```python
from build123d import *

# Parameters (mm, degrees)
SKETCH_1_R          = 34
EXTRUDE_1_DEPTH     = 29
SKETCH_2_R          = 25
CUT_EXTRUDE_1_DEPTH = 5
CUT_EXTRUDE_START   = -5
SKETCH_3_R          = 25
CUT_EXTRUDE_2_DEPTH = 5
CUT_EXTRUDE_3_DEPTH = 10
SKETCH_5_R          = 1.4
CUT_EXTRUDE_4_DEPTH = 54.74011537


with BuildPart() as part:
    # 草图1 → 凸台-拉伸1 (new body)
    with BuildSketch(Plane.XY):
        with Locations(Location((0, 0, 0), (0, 0, 180))):
            Circle(SKETCH_1_R)
    extrude(amount=EXTRUDE_1_DEPTH)

    # 草图2 → 切除-拉伸1 (cut)
    with BuildSketch(Plane.XY.offset(29)):
        Circle(SKETCH_2_R)
    extrude(amount=-CUT_EXTRUDE_1_DEPTH, mode=Mode.SUBTRACT)

    # 草图3 → 切除-拉伸2 (cut)
    with BuildSketch(Plane(origin=(0, 0, 0), x_dir=(-1, 0, 0), z_dir=(0, 0, -1)).offset(CUT_EXTRUDE_START)):
        with Locations(Location((0, 0, 0), (0, 0, 180))):
            Circle(SKETCH_3_R)
    extrude(amount=CUT_EXTRUDE_2_DEPTH, mode=Mode.SUBTRACT)

    # 草图4 → 切除-拉伸3 (cut)
    with BuildSketch(Plane(origin=(0, 0, 5), x_dir=(-1, 0, 0), z_dir=(0, 0, -1))):
        Polygon((2.352778868, -3.142891174), (3.898213032, 0.466120682), (1.545434164, 3.609011856), (-2.352778868, 3.142891174), (-3.898213032, -0.466120682), (-1.545434164, -3.609011856), align=None)
    extrude(amount=-CUT_EXTRUDE_3_DEPTH, mode=Mode.SUBTRACT)

    # 草图5 → 切除-拉伸4 (cut, through all)
    with BuildSketch(Plane.XY.offset(24)):
        Circle(SKETCH_5_R)
    extrude(amount=-CUT_EXTRUDE_4_DEPTH, mode=Mode.SUBTRACT)


solid = part.part
```
The listing builds one solid part. Answer for the finished solid, in the listing's coordinates (mm). A direction names the side the tool comes from. Give positions to 0.01 mm unless a question says otherwise; leave off trailing zeros. Order: outer loops, then holes, each group sorted by start corner. A loop starts at its lowest first (then second) coordinate and runs counter-clockwise, first axis right, second up. Notation, with made-up numbers: (89.25, 9.5) -> (140.25, 9.5) arc R12 ccw to (140.25, 28.5) -> close; hole circle Ø10 at (-24.5, 21.5). An arc over 180 degrees is marked (long way). One line per item, written item: value.
1) Find the intervals of material crossed by line 1 (Y direction, x = 0, z = 20.25); line 2 (Y direction, x = 0, z = 3.9); line 3 (Z direction, x = -15, y = 1), in increasing order.
Reported:
line 1: y = -34 to -1.4, 1.4 to 34
line 2: y = -34 to -25, 25 to 34
line 3: z = 5 to 24
2) A tool of negligible diameter and unlimited length cuts with its end or side. For faces 1 (the flat face through (-2.738, 2.016, 9.93)), 2 (the cylindrical face through (23.846, 7.509, 26.535)), 3 (the cylindrical face through (-1.4, 0.06, 19.56)), from which of +Z, -Z, +X, -X, +Y, -Y can it reach the whole face along a straight path? Write none if from no direction.
Reported:
face 1: -Z
face 2: +Z
face 3: +Z, -Z
3) Find section D-D, the plane x = 16. Determine the outline of the cut face in (y, z).
Reported:
outline: (-30, 0) -> (-19.21, 0) -> (-19.21, 5) -> (19.21, 5) -> (19.21, 0) -> (30, 0) -> (30, 29) -> (19.21, 29) -> (19.21, 24) -> (-19.21, 24) -> (-19.21, 29) -> (-30, 29) -> close
4) Find section A-A, the plane z = 12. Determine the outline of the cut face in (x, y).
Reported:
outline: circle Ø68 at (0, 0); hole (-3.9, 0.47) -> (-2.35, -3.14) -> (1.55, -3.61) -> (3.9, -0.47) -> (2.35, 3.14) -> (-1.55, 3.61) -> close
5) Flat-ended cylindrical pins translate along their axes: P1, Ø2, axis at y = -27, z = 5, coming from the +X side; P2, Ø8, axis at x = -22, z = 16, coming from the +Y side; P3, Ø1, axis at y = 22.5, z = 24, coming from the +X side. Find the tip coordinate at first contact, or state that the pin passes through.
Reported:
P1: stops at x = 21.91
P2: stops at y = 28.84
P3: stops at x = 25.92
6) Find section B-B, the plane x = 0. Determine the outline of the cut face in (y, z).
Reported:
outline: (-34, 0) -> (-25, 0) -> (-25, 5) -> (-3.42, 5) -> (-3.42, 15) -> (-1.4, 15) -> (-1.4, 24) -> (-25, 24) -> (-25, 29) -> (-34, 29) -> close; (1.4, 15) -> (3.42, 15) -> (3.42, 5) -> (25, 5) -> (25, 0) -> (34, 0) -> (34, 29) -> (25, 29) -> (25, 24) -> (1.4, 24) -> close
7) Find section C-C, the plane y = 12. Determine the outline of the cut face in (x, z).
Reported:
outline: (-31.81, 0) -> (-21.93, 0) -> (-21.93, 5) -> (21.93, 5) -> (21.93, 0) -> (31.81, 0) -> (31.81, 29) -> (21.93, 29) -> (21.93, 24) -> (-21.93, 24) -> (-21.93, 29) -> (-31.81, 29) -> close
8) Determine the mould class of faces 4 (the flat face through (0, -5, 24)), 5 (the flat face through (18, -18, 29)), 6 (the cylindrical face through (4.43, -33.71, 14.3)), 7 (the flat face through (0.38, 3.38, 9.93)) for opening direction X: pulls with the +X half, pulls with the -X half, needs draft (parallel to the pull), parting line crosses it, or undercut.
Reported:
face 4: undercut
face 5: needs draft
face 6: parting line crosses it
face 7: undercut
